The drawing under review shows one solid part. Ordinate dimensions are in mm from its lowest x, y, z. Coordinates: 2 decimals unless noted, no trailing zeros. Write each loop counter-clockwise with the first axis right and the second up, starting at its lowest first coordinate (ties: lowest second). Pieces come first, ordered by that corner, then holes. Notation, with made-up numbers: M -25.75,42.5 L -13.75,42.5 A25 cw -13.75,67.5 Z; hole C 18,10.25 d7. An arc over 180 degrees is marked long. Write item = value, one per line.
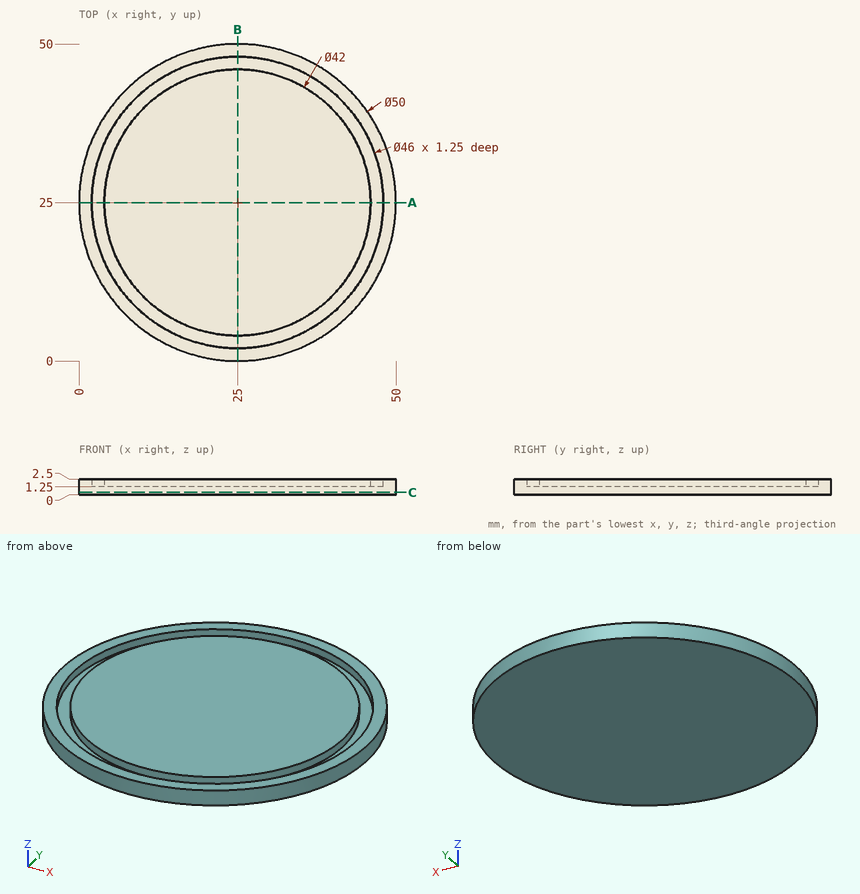
Q1. Consider section C-C, the plane z = 0.4. State the section outline as (x, y) points, and give its area (3 significant figures).
Check result:
outline = C 25,25 d50
area = 1,960 mm²
Q2. Wall thickness on line 1 (X direction, y = 24.5, z = 1.35) (3 decimals); line 2 (Y direction, x = 25, z = 1.6); line 3 (Y direction, x = 17.5, z = 2.3): over which ranges is each line inside the solid? List them lowest first.
Check result:
line_1 = 0.005 to 2.005, 4.006 to 45.994, 47.995 to 49.995
line_2 = 0 to 2, 4 to 46, 48 to 50
line_3 = 1.15 to 3.26, 5.38 to 44.62, 46.74 to 48.85
Q3. For P1, Ø1, axis at y = 26, z = 1.5, coming from the +X side (3 decimals), flat-tipped, find the tip position at first contact; note if it passes through.
Check result:
P1 = 49.995
Q4. Consider section A-A, the plane y = 25. State the section outline as (x, z) points.
Check result:
outline = M 0,0 L 50,0 L 50,2.5 L 48,2.5 L 48,1.25 L 46,1.25 L 46,2.5 L 4,2.5 L 4,1.25 L 2,1.25 L 2,2.5 L 0,2.5 Z
